Check sheet for the modelled part. Datum: model origin and axes. Units: mm. Round coordinates to 2 decimals unless told otherwise and drop trailing zeros. Write each loop counter-clockwise with the first axis right and the second up, starting at its lowest first coordinate (ties: lowest second). Pieces come first, ordered by that corner, then holes. Notation, with made-up numbers: M 80,-29 L 91,-29 A32 cw 91,0 Z; hole C 49.25,44.5 d11. An arc over 180 degrees is marked long. One line per item, written item: value.
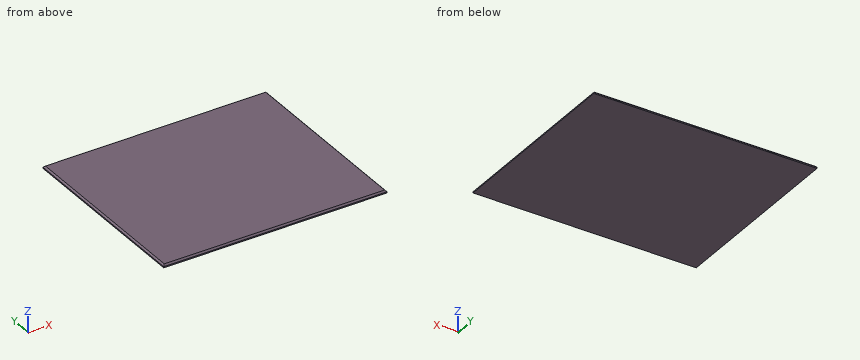
from build123d import *

# Parameters (mm, degrees)
F0_W     = 44.8449254036
F0_H     = 43.0354773998
F1_DEPTH = 7
F2_DEPTH = 590
F3_DEPTH = 500
F4_SIZE  = 4


with BuildPart() as f1:
    # F0 (on Top) → F1 (new body)
    with BuildSketch(Plane.XY):
        with Locations((22.4224627018, 21.5177386999)):
            Rectangle(F0_W, F0_H)
    extrude(amount=F1_DEPTH)

    # F2 (add): a face of the model
    f2_faces = [f1.faces().sort_by_distance(p)[0] for p in [
        (0, 21.5177386999, 3.5),
    ]]
    extrude(f2_faces, amount=-F2_DEPTH)

    # F3 (add): a face of the model
    f3_faces = [f1.faces().sort_by_distance(p)[0] for p in [
        (295, 0, 3.5),
    ]]
    extrude(f3_faces, amount=-F3_DEPTH)

    # F4
    f4_edges = [f1.edges().sort_by_distance(p)[0] for p in [
        (0, 250, 7),
        (295, 0, 7),
        (590, 250, 7),
        (295, 500, 7),
    ]]
    chamfer(f4_edges, length=F4_SIZE)


solid = f1.part
Q1. Sectioned sample at A-A on z = 5.5. Enter the section's corners in (x, y).
Completed:
outline: M 2.5,2.5 L 587.5,2.5 L 587.5,497.5 L 2.5,497.5 Z
Q2. Scan lines: line 1 (Y direction, x = 212, z = 6.5); line 2 (Y direction, x = 309, z = 6.25); line 3 (X direction, y = 202, z = 5.75). Record each from-to range of solid material in increasing order. Write a range as [from, to].
Completed:
line 1: [3.5, 496.5]
line 2: [3.25, 496.75]
line 3: [2.75, 587.25]
Q3. Depth check by flat-ended pin: P1, Ø3, axis at x = 450, z = 5.5, coming from the -Y side. Enter the tip coordinate at first touch or a pass-through.
Completed:
P1: y = 1
